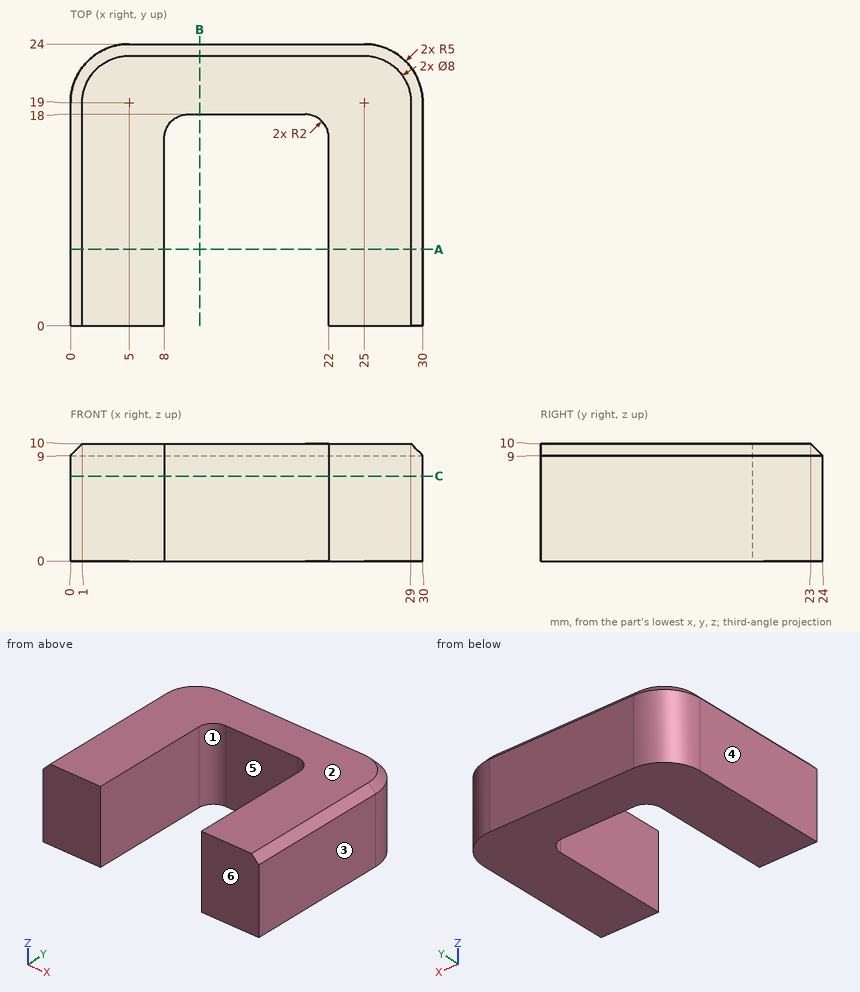
Input: dimensioned drawing with shaded views. Units: mm. Origin: part minimum x, y, z. A direction names the side the tool comes from. Give positions to 0.01 mm unless a question says otherwise; leave off trailing zeros. Write each loop counter-clockwise with the first axis right and the second up, starting at its lowest first coordinate (ties: lowest second). Pieces come first, ordered by that corner, then holes. Notation, with made-up numbers: M 35,45.5 L 71,45.5 A33 ccw 71,77.5 Z; hole C 42.5,5.25 d1. An arc over 180 degrees is marked long. Return JSON: item names as keys, results as strings. Group by question number.
1) Pin query (flat end, axial travel): P1, Ø6, axis at x = 5, y = 3, coming from the -Z side. Return the tip coordinate at first contact, or that it passes through.
2) Cut plane A-A, the plane y = 6.5. Output: boundary loops of the cut face in (x, z).
3) Cut plane C-C, the plane z = 7.25. Output: boundary loops of the cut face in (x, y), plus the area to 3 significant figures.
4) Material intervals for line 1 along X through (y, z) = (11.25, 5.75); line 2 along Y through (x, z) = (9, 5.5); line 3 along X through (y, z) = (20.75, 5.75), sorted ascending. Write a range as [from, to].
5) Cut plane B-B, the plane x = 11. Output: boundary loops of the cut face in (y, z).
6) Pull-direction query (X, two-part tool) for the marked faces 3, 4, 5 and 6; classes: pulls with the +X half, pulls with the -X half, needs draft (parallel to the pull), parting line crosses it, or undercut.
7) Set-up query: the marked faces 1 and 2. Return all of +Z, -Z, +X, -X, +Y, -Y with unobstructed straight access to the full face (end or side cutting, diameter ignored); none if empty.
Recorded:
{
 "1": {"P1": "stops at z = 0"},
 "2": {"outline": "M 0,0 L 8,0 L 8,10 L 1,10 L 0,9 Z; M 22,0 L 30,0 L 30,9 L 29,10 L 22,10 Z"},
 "3": {"outline": "M 0,0 L 8,0 L 8,16 A2 cw 10,18 L 20,18 A2 cw 22,16 L 22,0 L 30,0 L 30,19 A5 ccw 25,24 L 5,24 A5 ccw 0,19 Z", "area": "459 mm²"},
 "4": {"line 1": "x = [0, 8], [22, 30]", "line 2": "y = [17.73, 24]", "line 3": "x = [0.32, 29.68]"},
 "5": {"outline": "M 18,0 L 24,0 L 24,9 L 23,10 L 18,10 Z"},
 "6": {"face 3": "pulls with the +X half", "face 4": "pulls with the -X half", "face 5": "undercut", "face 6": "needs draft"},
 "7": {"face 1": "+Z, -Z, -Y", "face 2": "+Z, +X, -X, +Y, -Y"}
}
